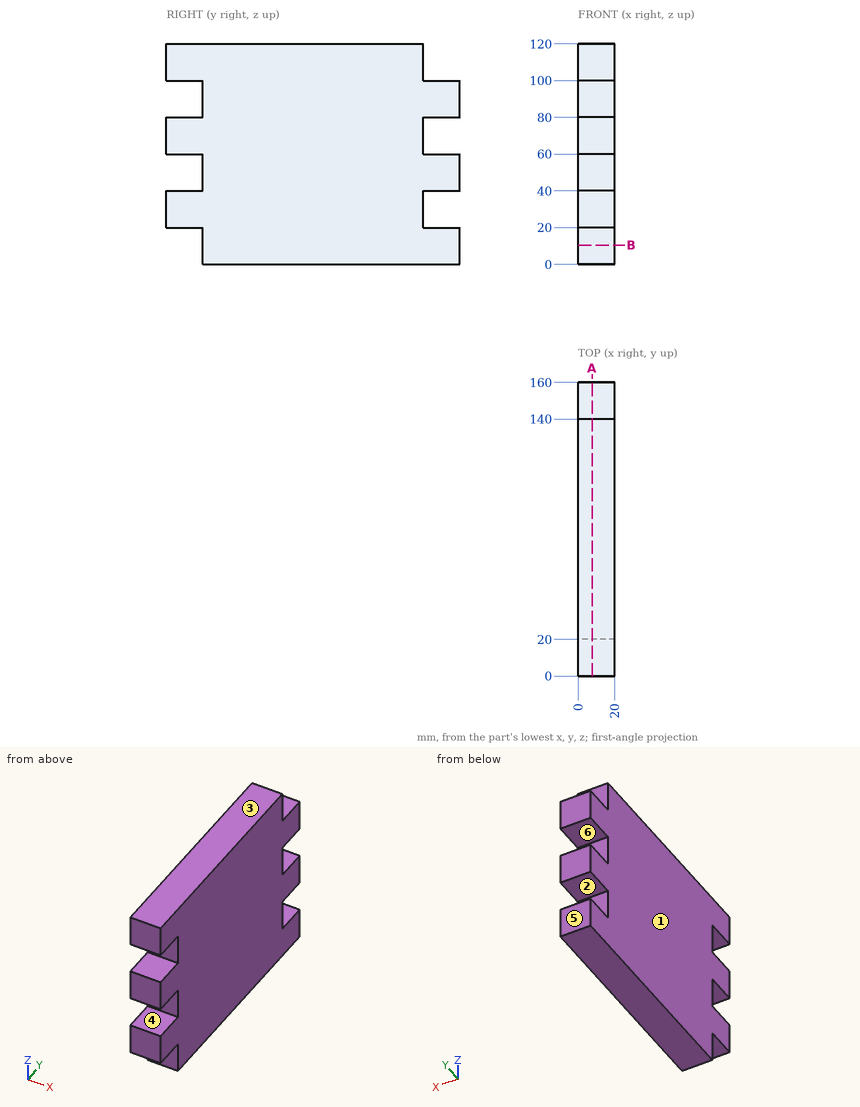
Check sheet for the drawn part. Datum: minimum x, y, z corner. Units: mm. A direction names the side the tool comes from. Coordinates: 2 decimals unless noted, no trailing zeros. Loops run counter-clockwise (first coordinate to the right, second up) from the corner with the lowest first, then second, coordinate; pieces in that order, holes last. Notation, with made-up numbers: (-28.5, -40) -> (13.5, -40) arc R21 cw to (13.5, -36) -> close; hole circle Ø8 at (31, 78.25). An arc over 180 degrees is marked (long way). Answer as CSV lines item,"result".
1) Cross-section at A-A, the plane x = 7.75. Record the cut outline in (y, z).
Found:
outline,"(0, 20) -> (20, 20) -> (20, 0) -> (160, 0) -> (160, 20) -> (140, 20) -> (140, 40) -> (160, 40) -> (160, 60) -> (140, 60) -> (140, 80) -> (160, 80) -> (160, 100) -> (140, 100) -> (140, 120) -> (0, 120) -> (0, 100) -> (20, 100) -> (20, 80) -> (0, 80) -> (0, 60) -> (20, 60) -> (20, 40) -> (0, 40) -> close"
2) Tool access check on the marked faces 4, 5 and 6. Record the directions out of +Z, -Z, +X, -X, +Y, -Y that give a thin tool (end or side, any length) a straight path to the whole face; none if there is none.
Found:
face 4,"+X, -X, -Y"
face 5,"+Z, -Z, +X, -X, +Y"
face 6,"+X, -X, +Y"
3) Thickness scan on L1, parallel to Z at x = 10.5, y = 145; L2, parallel to Y at x = 19.25, z = 11; L3, parallel to Y at x = 5.5, z = 29.5. Record the ranges inside material, lowest first. Write a range as from..to.
Found:
L1,"z = 0..20, 40..60, 80..100"
L2,"y = 20..160"
L3,"y = 0..140"
4) Cross-section at B-B, the plane z = 10.5. Record the cut outline in (x, y).
Found:
outline,"(0, 20) -> (20, 20) -> (20, 160) -> (0, 160) -> close"
5) Depth check by flat-ended pin: pin 1 (1.5 mm diameter, centred on x = 11, z = 19, fed in from -Y); pin 2 (10 mm diameter, centred on x = 10, y = 9, fed in from -Z); pin 3 (10 mm diameter, centred on x = 14, z = 79.5, fed in from -Y); pin 4 (1 mm diameter, centred on x = 14.5, z = 102, fed in from +Y). Enter the tip coordinate at first touch or a pass-through.
Found:
pin 1,"stops at y = 20"
pin 2,"stops at z = 20"
pin 3,"stops at y = 0"
pin 4,"stops at y = 140"
6) Release check for a two-part mould opening along Z. For the marked faces 1, 2 and 3 record: +Z half, -Z half, draft (parallel to the pull), parting line (faces both ways), or undercut.
Found:
face 1,"draft"
face 2,"undercut"
face 3,"+Z half"
